```python
from build123d import *

# Parameters (mm, degrees)
F0_R     = 50.8
F1_DEPTH = 25.4
F2_R     = 5.08
F3_R     = 6.35
F4_DEPTH = 25.401


with BuildPart() as f1:
    # F0 (on Front) → F1 (new body)
    with BuildSketch(Plane.XZ):
        Circle(F0_R)
    extrude(amount=F1_DEPTH)

    # F2
    f2_edges = [f1.edges().sort_by_distance(p)[0] for p in [
        (-50.8, -25.4, 0),
        (-50.8, 0, 0),
    ]]
    fillet(f2_edges, radius=F2_R)

    # F3 (on face) → F4 (cut, through all)
    with BuildSketch(Plane.XZ.offset(25.4)):
        Circle(F3_R)
    extrude(amount=-F4_DEPTH, mode=Mode.SUBTRACT)


solid = f1.part
```
Verification items for the finished model (mm, model axes). Give positions to 0.01 mm unless a question says otherwise; leave off trailing zeros. Loops run counter-clockwise (first coordinate to the right, second up) from the corner with the lowest first, then second, coordinate; pieces in that order, holes last. Notation, with made-up numbers: M 72,70.25 L 87,70.25 A34 cw 87,104.25 Z; hole C 57,28 d3. An arc over 180 degrees is marked long. One line per question, with ' | ' between items.
Item 1: Section check A-A, the plane x = 0. Record the cut outline in (y, z).
Completed:
outline: M -25.4,-45.72 A5.08 ccw -20.32,-50.8 L -5.08,-50.8 A5.08 ccw 0,-45.72 L 0,-6.35 L -25.4,-6.35 Z; M -25.4,6.35 L 0,6.35 L 0,45.72 A5.08 ccw -5.08,50.8 L -20.32,50.8 A5.08 ccw -25.4,45.72 Z
Item 2: Section check B-B, the plane z = 0. Record the cut outline in (x, y).
Completed:
outline: M -50.8,-20.32 A5.08 ccw -45.72,-25.4 L -6.35,-25.4 L -6.35,0 L -45.72,0 A5.08 ccw -50.8,-5.08 Z; M 6.35,-25.4 L 45.72,-25.4 A5.08 ccw 50.8,-20.32 L 50.8,-5.08 A5.08 ccw 45.72,0 L 6.35,0 Z
Item 3: Section check C-C, the plane y = -11.5. Record the cut outline in (x, z).
Completed:
outline: C 0,0 d101.6; hole C 0,0 d12.7
Item 4: Draft check along X on faces 1 (the face through (-1.38, -12.88, -6.2)), 2 (the face through (-1, 0, -10)), 3 (the face through (-11.012, -12.593, -49.592)). Enter one of: +X half, -X half, draft (parallel to the pull), parting line (faces both ways), or undercut.
Completed:
face 1: undercut | face 2: draft | face 3: parting line
Item 5: Depth check by flat-ended pin: P1, Ø1.5, axis at x = -40.5, z = 24.5, coming from the -Y side; P2, Ø6, axis at y = -17, z = 8.5, coming from the -X side; P3, Ø4, axis at x = -32, y = -17, coming from the -Z side. Enter the tip coordinate at first touch or a pass-through.
Completed:
P1: stops at y = -25.33 | P2: stops at x = -50.5 | P3: stops at z = -41
Item 6: Thickness scan on line 1 (Z direction, x = 0, y = -17); line 2 (X direction, y = -9, z = -1); line 3 (X direction, y = -11.5, z = -9). Record the ranges inside material, lowest first. Write a range as [from, to].
Completed:
line 1: z = [-50.8, -6.35], [6.35, 50.8] | line 2: x = [-50.79, -6.27], [6.27, 50.79] | line 3: x = [-50, 50]
